from build123d import *

# Parameters (mm, degrees)
ESQUISSE1_R             = 46
BOSS_EXTRU_1_DEPTH      = 3
ESQUISSE2_R             = 46
BOSS_EXTRU_2_DEPTH      = 5
BOSS_EXTRU_2_TAPER      = 75
ESQUISSE3_R             = 2
ENL_V_MAT_EXTRU_1_DEPTH = 66.543878433
ESQUISSE4_R             = 14
ENL_V_MAT_EXTRU_2_DEPTH = 66.543878433
CHANFREIN1_SIZE         = 0.5
CHANFREIN1_SIZE2        = 0.714074003


# Read off the part's stored shape, not the designer's step: Coque1
with BuildPart() as part:
    # Esquisse1 → Boss.-Extru.1 (new body)
    with BuildSketch(Plane.XY):
        Circle(ESQUISSE1_R)
    extrude(amount=BOSS_EXTRU_1_DEPTH)

    # Esquisse2 → Boss.-Extru.2 (add)
    with BuildSketch(Plane.XY.offset(3)):
        Circle(ESQUISSE2_R)
    extrude(amount=BOSS_EXTRU_2_DEPTH, taper=BOSS_EXTRU_2_TAPER)

    # Coque1 outline → Coque1 (revolve, cut)
    with BuildSketch(Plane.XZ):
        Polygon((37.877635897, 0), (26.681483474, 3), (0, 3), (0, 0), align=None)
    revolve(axis=Axis((0, 0, 0), (0, 0, 1)), mode=Mode.SUBTRACT)

    # Esquisse3 → Enlèv. mat.-Extru.1 (cut, through all)
    with BuildSketch(Plane.XY.offset(8)):
        with Locations((0, 20)):
            Circle(ESQUISSE3_R)
        with Locations((20, 0)):
            Circle(ESQUISSE3_R)
        with Locations((0, -20)):
            Circle(ESQUISSE3_R)
        with Locations((-20, 0)):
            Circle(ESQUISSE3_R)
    extrude(amount=-ENL_V_MAT_EXTRU_1_DEPTH, mode=Mode.SUBTRACT)

    # Esquisse4 → Enlèv. mat.-Extru.2 (cut, through all)
    with BuildSketch(Plane.XY.offset(8)):
        Circle(ESQUISSE4_R)
    extrude(amount=-ENL_V_MAT_EXTRU_2_DEPTH, mode=Mode.SUBTRACT)

    # Chanfrein1
    chanfrein1_edges = [part.edges().sort_by_distance(p)[0] for p in [
        (-2, 20, 8),
        (18, 0, 8),
        (-2, -20, 8),
        (-22, 0, 8),
    ]]
    chanfrein1_side = [part.faces().sort_by_distance(p)[0] for p in [
        (-26.566461172, 0, 8),
    ]]
    chamfer(chanfrein1_edges, length=CHANFREIN1_SIZE, length2=CHANFREIN1_SIZE2, reference=chanfrein1_side[0])


solid = part.part
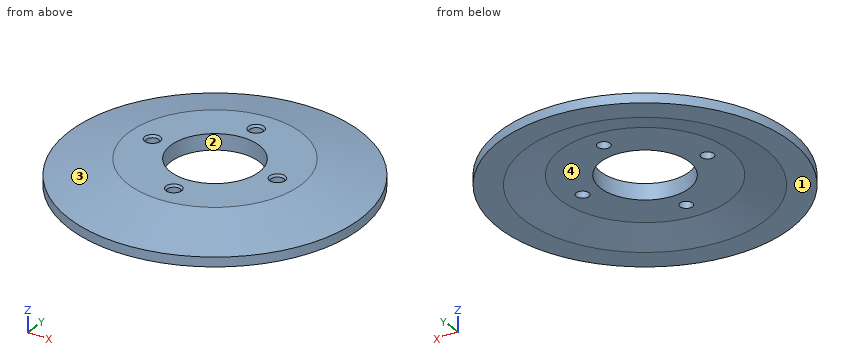
Can you work these out from the model? Positions are in its coordinate system, mm. Face numbers are marked on the shaded views. Coordinates: 2 decimals unless noted, no trailing zeros. Write each loop counter-clockwise with the first axis right and the second up, starting at its lowest first coordinate (ties: lowest second). Pieces come first, ordered by that corner, then holes. Notation, with made-up numbers: (-16, -20) - (19, -20) arc R18 ccw to (19, 15) - close; hole circle Ø9 at (86.5, 58). An arc over 180 degrees is marked (long way). Return JSON: item names as keys, results as strings. Group by question number.
Item 1: Please list where these lines run through material, in increasing order: probe 1 along Z at (x, y) = (4, -14); probe 2 along Z at (x, y) = (2, 33.5); probe 3 along Y at (x, z) = (41, 1).
Item 2: If we section it at A-A (x = 0): Write out the boundary of the cut face in (y, z), then the cut area to 3 significant figures.
Item 3: I'm going to push flat-ended pins straight in: pin 1 Ø8 at (x, y) = (17.5, -25) entering from -Z; pin 2 Ø6.5 at (x, y) = (0, 20) entering from -Z; pin 3 Ø3 at (x, y) = (24, 31) entering from +Z. Where does each tip first touch, or does it pass through?
Item 4: We'd pull the mould along Y, two halves only. Please class the marked faces 1, 2, 3 and 4: pulls with the +Y half, pulls with the -Y half, needs draft (parallel to the pull), parting line crosses it, or undercut.
Return value:
{
 "1": {"probe 1": "z = 3 to 8", "probe 2": "z = 1.16 to 6.33", "probe 3": "y = -20.86 to 20.86"},
 "2": {"outline": "(-46, 0) - (-37.88, 0) - (-26.68, 3) - (-22, 3) - (-22, 7.29) - (-22.5, 8) - (-27.34, 8) - (-46, 3) - close; (-18, 3) - (-14, 3) - (-14, 8) - (-17.5, 8) - (-18, 7.29) - close; (14, 3) - (18, 3) - (18, 7.29) - (17.5, 8) - (14, 8) - close; (22, 3) - (26.68, 3) - (37.88, 0) - (46, 0) - (46, 3) - (27.34, 8) - (22.5, 8) - (22, 7.29) - close", "area": "268 mm^2"},
 "3": {"pin 1": "stops at z = 0.9", "pin 2": "stops at z = 3", "pin 3": "stops at z = 5.22"},
 "4": {"face 1": "needs draft", "face 2": "undercut", "face 3": "parting line crosses it", "face 4": "undercut"}
}
